Geometry: see drawing. Coordinates: mm, zero at the bounding-box minimum. A direction names the side the tool comes from. Round coordinates to 2 decimals unless told otherwise and drop trailing zeros. Loops run counter-clockwise (first coordinate to the right, second up) from the corner with the lowest first, then second, coordinate; pieces in that order, holes last. Notation, with made-up numbers: (-4.5, 82) - (0.5, 82) arc R18 ccw to (0.5, 96) - close; hole circle Ø2 at (12.5, 50). An arc over 180 degrees is marked (long way). One line per question, with ' | ' between items. Start each with the question number.
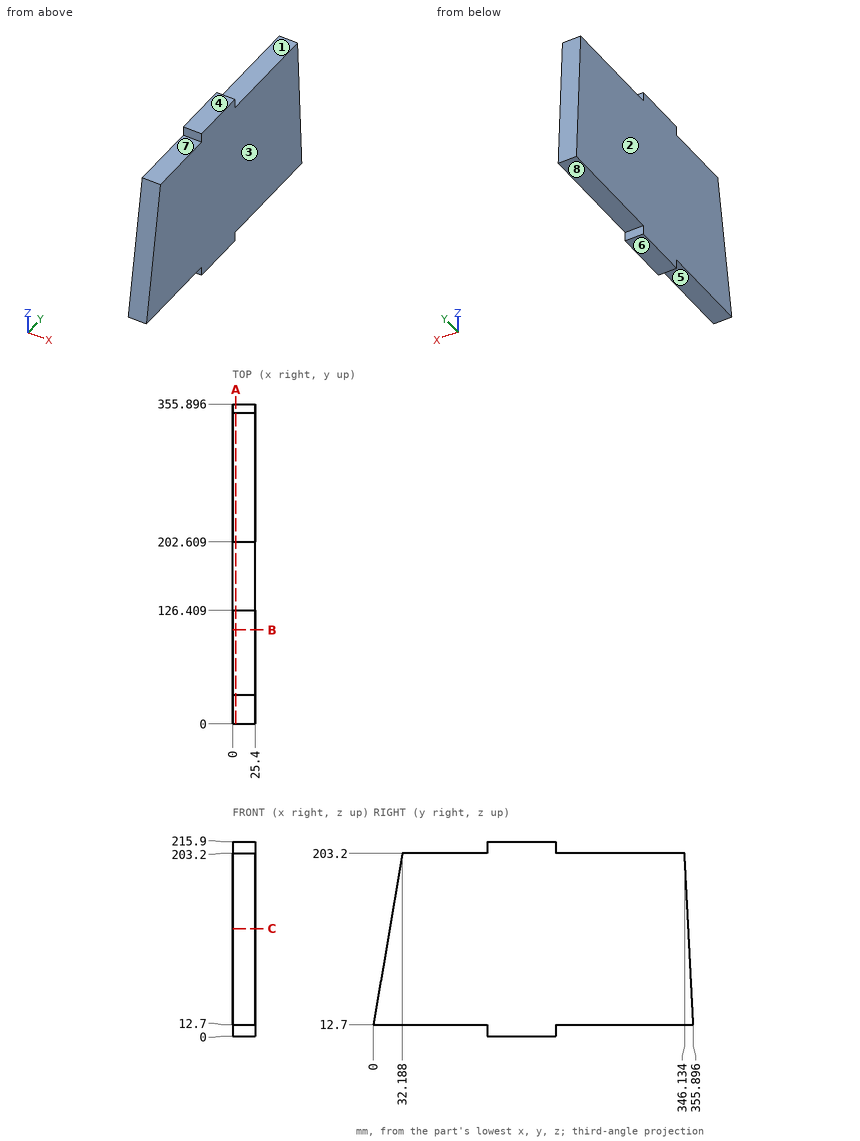
(1) Line query: line 1 along Z through (x, y) = (6.25, 316); line 2 along Y through (x, z) = (7, 12); line 3 along Y through (x, z) = (9.5, 145) (1 decimal). Output: solid intervals per line, ascending. Write a range as from..to.
(2) Section C-C, the plane z = 119.5. Output: boundary loops of the cut face in (x, y) (1 decimal), plus the area to 3 significant figures.
(3) Section A-A, the plane x = 3.5. Output: boundary loops of the cut face in (y, z).
(4) Pull-direction query (X, two-part tool) for the marked faces 1, 2 and 3; classes: released by +X, released by -X, zero draft, split by the parting line, or undercut.
(5) Section B-B, the plane y = 104.5. Output: boundary loops of the cut face in (x, z), plus the area to 3 significant figures.
(6) Reachability of the marked faces 4, 5, 6, 7 and 8 from +Z, -Z, +X, -X, +Y, -Y: full face, straight path, thin tool, end or side. Return the list, or none.
(7) Pin query (flat end, axial travel): P1, Ø5, axis at x = 21.5, y = 310, coming from the +Z side; P2, Ø12.5, axis at x = 15, y = 52.5, coming from the -Z side; P3, Ø6.5, axis at x = 13, z = 4, coming from the +Y side. Return the tip coordinate at first contact, or that it passes through.
Derived:
1) line 1: z = 12.7..203.2 | line 2: y = 126.41..202.61 | line 3: y = 22.4..349.1
2) outline: (0, 18) - (25.4, 18) - (25.4, 350.4) - (0, 350.4) - close | area: 8,440 mm²
3) outline: (0, 12.7) - (126.41, 12.7) - (126.41, 0) - (202.61, 0) - (202.61, 12.7) - (355.9, 12.7) - (346.13, 203.2) - (202.61, 203.2) - (202.61, 215.9) - (126.41, 215.9) - (126.41, 203.2) - (32.19, 203.2) - close
4) face 1: zero draft | face 2: released by -X | face 3: released by +X
5) outline: (0, 12.7) - (25.4, 12.7) - (25.4, 203.2) - (0, 203.2) - close | area: 4,840 mm²
6) face 4: +Z, +X, -X, +Y, -Y | face 5: -Z, +X, -X, -Y | face 6: -Z, +X, -X, +Y, -Y | face 7: +Z, +X, -X, -Y | face 8: -Z, +X, -X, +Y
7) P1: stops at z = 203.2 | P2: stops at z = 12.7 | P3: stops at y = 202.61
